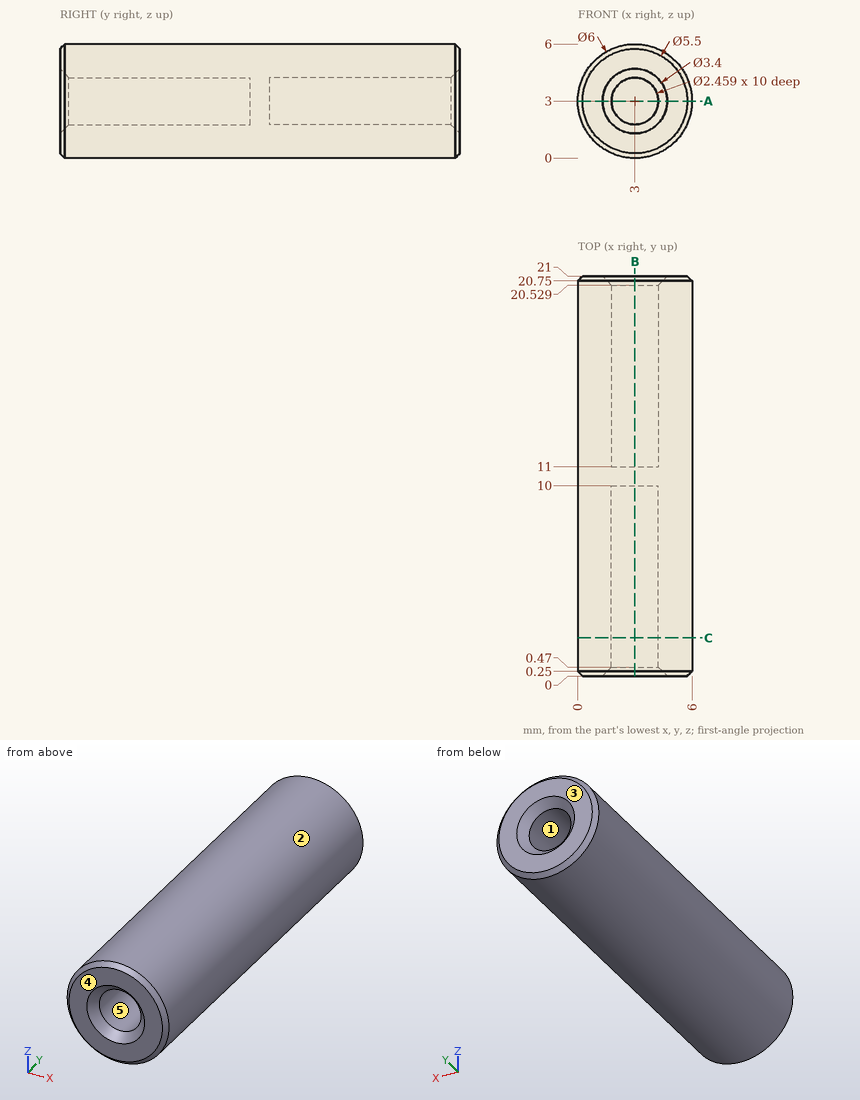
Check sheet for the drawn part. Datum: minimum x, y, z corner. Units: mm. A direction names the side the tool comes from. Coordinates: 2 decimals unless noted, no trailing zeros. Order: outer loops, then holes, each group sorted by start corner. A loop starts at its lowest first (then second) coordinate and runs counter-clockwise, first axis right, second up. Notation, with made-up numbers: (-40, -37.5) -> (12, -37.5) arc R27 ccw to (12, -18.5) -> close; hole circle Ø9 at (-8.75, 57.25). An arc over 180 degrees is marked (long way). Use a Markdown table: item, result. Add a question column.
1. Set-up check for the marked faces 4 and 5: record each of +Z, -Z, +X, -X, +Y, -Y from which the full face is reachable in a straight line by a thin tool's end or side.
2. Cross-section at A-A (z = 3). Enter the section's corners in (x, y).
3. Cross-section at B-B (x = 3). Enter the section's corners in (y, z).
4. Mould release check, pull along Z, two halves, no side actions. Record for the marked faces 1, 2 and 3: pulls with the +Z half, pulls with the -Z half, needs draft (parallel to the pull), parting line crosses it, or undercut.
5. Go/stop test with flat-tipped pins: pin 1 Ø0.7 at (x, z) = (3.5, 3) entering from +Y; pin 2 Ø3 at (y, z) = (16.5, 4) entering from +X; pin 3 Ø3 at (x, z) = (3, 3) entering from +Y; pin 4 Ø1 at (y, z) = (3.5, 1) entering from +X. Record where each tip stops, or that it passes through.
6. Material ranges on L1, parallel to Z at x = 3, y = 6.75; L2, parallel to Z at x = 3.45, y = 16.75 (1 decimal); L3, parallel to X at y = 14.5, z = 2.75 (1 decimal), recorded low to high.
7. Cross-section at C-C (y = 2). Enter the section's corners in (x, z).
Filled sheet:
| question | item | result |
|---|---|---|
| 1 | face 4 | +Z, -Z, +X, -X, -Y |
| 1 | face 5 | -Y |
| 2 | outline | (0, 0.25) -> (0.25, 0) -> (1.3, 0) -> (1.77, 0.47) -> (1.77, 10) -> (4.23, 10) -> (4.23, 0.47) -> (4.7, 0) -> (5.75, 0) -> (6, 0.25) -> (6, 20.75) -> (5.75, 21) -> (4.7, 21) -> (4.23, 20.53) -> (4.23, 11) -> (1.77, 11) -> (1.77, 20.53) -> (1.3, 21) -> (0.25, 21) -> (0, 20.75) -> close |
| 3 | outline | (0, 0.25) -> (0.25, 0) -> (20.75, 0) -> (21, 0.25) -> (21, 1.3) -> (20.53, 1.77) -> (11, 1.77) -> (11, 4.23) -> (20.53, 4.23) -> (21, 4.7) -> (21, 5.75) -> (20.75, 6) -> (0.25, 6) -> (0, 5.75) -> (0, 4.7) -> (0.47, 4.23) -> (10, 4.23) -> (10, 1.77) -> (0.47, 1.77) -> (0, 1.3) -> close |
| 4 | face 1 | undercut |
| 4 | face 2 | parting line crosses it |
| 4 | face 3 | needs draft |
| 5 | pin 1 | y = 11 |
| 5 | pin 2 | x = 6 |
| 5 | pin 3 | y = 20.8 |
| 5 | pin 4 | x = 5.6 |
| 6 | L1 | 0 to 1.77, 4.23 to 6 |
| 6 | L2 | 0 to 1.9, 4.1 to 6 |
| 6 | L3 | 0 to 1.8, 4.2 to 6 |
| 7 | outline | circle Ø6 at (3, 3); hole circle Ø2.46 at (3, 3) |
